```python
from build123d import *

# Parameters (mm, degrees)
F0_W      = 76.2
F0_H      = 76.2
F1_DEPTH  = 19.05
F2_R      = 25.4
F3_DEPTH  = 76.2
F5_W      = 76.2
F5_H      = 76.2
F5_R      = 25.4
F4_R      = 25.4
F6_DEPTH  = 19.05
F8_DEPTH  = 114.301
F9_R      = 6.35
F10_R     = 6.35
F11_DEPTH = 25.4
F12_R     = 6.35
F13_DEPTH = 114.301


with BuildPart() as f1:
    # F0 (on Front) → F1 (new body)
    with BuildSketch(Plane.XZ):
        with Locations((0, -0.0663684971)):
            Rectangle(F0_W, F0_H)
    extrude(amount=F1_DEPTH)

    # F2 (on face) → F3 (join)
    with BuildSketch(Plane.XZ.offset(19.05)):
        Circle(F2_R)
    extrude(amount=F3_DEPTH)

    # F5 (on face) + F4 (on face) → F6 (join)
    with BuildSketch(Plane.XZ.offset(95.25)):
        with Locations((-0.1962948591, 0.8762047957)):
            Rectangle(F5_W, F5_H)
        Circle(F5_R, mode=Mode.SUBTRACT)
    with BuildSketch(Plane.XZ.offset(95.25)):
        Circle(F4_R)
    extrude(amount=F6_DEPTH)

    # F7 (on face) → F8 (cut, through all)
    with BuildSketch(Plane.XZ.offset(114.3)):
        with BuildLine():
            Line((-0.196411438, 0.8763213746), (-13.1261387718, 13.8060487085))
            ThreePointArc((-13.1261387718, 13.8060487085), (-19.0399198266, 0.6196394072), (-13.9960272385, -12.9233788747))
            Line((-13.9960272385, -12.9233788747), (-0.196411438, 0.8763213746))
        make_face()
        with BuildLine():
            Line((13.8060487085, -13.1261387718), (-0.196411438, 0.8763213746))
            Line((-0.196411438, 0.8763213746), (-13.9960272385, -12.9233788747))
            ThreePointArc((-13.9960272385, -12.9233788747), (-0.1389275151, -19.0494934092), (13.8060487085, -13.1261387718))
        make_face()
        with BuildLine():
            Line((12.923293224, 13.9961063245), (-0.196411438, 0.8763213746))
            Line((-0.196411438, 0.8763213746), (13.8060487085, -13.1261387718))
            ThreePointArc((13.8060487085, -13.1261387718), (17.690502083, -7.067434899), (19.05, 0))
            ThreePointArc((19.05, 0), (17.4512354279, 7.6391676275), (12.923293224, 13.9961063245))
        make_face()
        with BuildLine():
            ThreePointArc((12.923293224, 13.9961063245), (-0.138985803, 19.049492984), (-13.1261387718, 13.8060487085))
            Line((-13.1261387718, 13.8060487085), (-0.196411438, 0.8763213746))
            Line((-0.196411438, 0.8763213746), (12.923293224, 13.9961063245))
        make_face()
    extrude(amount=-F8_DEPTH, mode=Mode.SUBTRACT)

    # F9 (on face) + F10 (on face) → F11 (cut)
    with BuildSketch(Plane.XZ.offset(114.3)):
        with Locations((28.3787051409, -27.6987952043)):
            Circle(F9_R)
        with Locations((-28.7712948591, 29.4512047957)):
            Circle(F9_R)
        with Locations((-28.7712948591, -27.6987952043)):
            Circle(F9_R)
    with BuildSketch(Plane.XZ.offset(114.3)):
        with Locations((28.3787051409, 29.4512047957)):
            Circle(F10_R)
    extrude(amount=-F11_DEPTH, mode=Mode.SUBTRACT)

    # F12 (on face) → F13 (cut, through all)
    with BuildSketch(Plane(origin=(0, 0, 0), x_dir=(-1, 0, 0), z_dir=(0, 1, 0))):
        with Locations((28.575, -28.6413684971)):
            Circle(F12_R)
        with Locations((28.575, 28.5086315029)):
            Circle(F12_R)
        with Locations((-28.575, 28.5086315029)):
            Circle(F12_R)
        with Locations((-28.575, -28.6247763728)):
            Circle(F12_R)
    extrude(amount=-F13_DEPTH, mode=Mode.SUBTRACT)


solid = f1.part
```
The listing builds one solid part. Answer for the finished solid, in the listing's coordinates (mm). A direction names the side the tool comes from. Give positions to 0.01 mm unless a question says otherwise; leave off trailing zeros. Order: outer loops, then holes, each group sorted by start corner. A loop starts at its lowest first (then second) coordinate and runs counter-clockwise, first axis right, second up. Notation, with made-up numbers: (50.25, 66.25) -> (81.25, 66.25) arc R28 cw to (81.25, 96.25) -> close; hole circle Ø3 at (-15.5, 20). An arc over 180 degrees is marked (long way). Write each question's results on one line, items separated by ' | '.
Q1. Straight lines are drawn through the part: probe 1 along Y at (x, z) = (26.5, -13.5); probe 2 along Z at (x, y) = (30.5, -8); probe 3 along Z at (x, y) = (3.5, -39). For each, find the intervals that lie inside material, in ascending order. Write a range as from..to.
Checked values:
probe 1: y = -114.3..-95.25, -19.05..0 | probe 2: z = -38.17..-34.68, -22.57..22.46, 34.56..38.03 | probe 3: z = -25.16..-18.73, 18.73..25.16
Q2. The part is cut by section B-B, the plane z = -6.5. Give the vertices of the cut face in (x, y).
Checked values:
outline: (-38.3, -114.3) -> (-17.91, -114.3) -> (-17.91, 0) -> (-38.1, 0) -> (-38.1, -19.05) -> (-24.55, -19.05) -> (-24.55, -95.25) -> (-38.3, -95.25) -> close; (17.91, -114.3) -> (37.9, -114.3) -> (37.9, -95.25) -> (24.55, -95.25) -> (24.55, -19.05) -> (38.1, -19.05) -> (38.1, 0) -> (17.91, 0) -> close
Q3. The part is cut by section D-D, the plane x = 29. Give the vertices of the cut face in (y, z), and give its area (3 significant figures).
Checked values:
outline: (-114.3, -37.22) -> (-95.25, -37.22) -> (-95.25, -34.96) -> (-114.3, -34.96) -> close; (-114.3, -21.38) -> (-95.25, -21.38) -> (-95.25, 22.17) -> (-114.3, 22.17) -> close; (-114.3, 35.77) -> (-95.25, 35.77) -> (-95.25, 38.98) -> (-114.3, 38.98) -> close; (-19.05, -38.17) -> (0, -38.17) -> (0, -34.96) -> (-19.05, -34.96) -> close; (-19.05, -22.29) -> (0, -22.29) -> (0, 22.17) -> (-19.05, 22.17) -> close; (-19.05, 34.84) -> (0, 34.84) -> (0, 38.03) -> (-19.05, 38.03) -> close | area: 1,900 mm^2
Q4. The part is cut by section A-A, the plane x = 0. Give the vertices of the cut face in (y, z).
Checked values:
outline: (-114.3, -37.22) -> (-95.25, -37.22) -> (-95.25, -25.4) -> (-19.05, -25.4) -> (-19.05, -38.17) -> (0, -38.17) -> (0, -19.05) -> (-114.3, -19.05) -> close; (-114.3, 19.05) -> (0, 19.05) -> (0, 38.03) -> (-19.05, 38.03) -> (-19.05, 25.4) -> (-95.25, 25.4) -> (-95.25, 38.98) -> (-114.3, 38.98) -> close
Q5. Determine the mould class of faces 1 (the face through (-9, 0, 17)), 2 (the face through (27.205, -104.908, -21.458)), 3 (the face through (-5.506, -56.617, -24.796)) for opening direction Y: pulls with the +Y half, pulls with the -Y half, needs draft (parallel to the pull), parting line crosses it, or undercut.
Checked values:
face 1: pulls with the +Y half | face 2: needs draft | face 3: undercut
Q6. The part is cut by section C-C, the plane y = -42.5. Give the vertices of the cut face in (x, z), and give its area (3 significant figures).
Checked values:
outline: circle Ø50.8 at (0, 0); hole circle Ø38.1 at (0, 0) | area: 887 mm^2
Q7. Each of these flat-tipped pins is pushed along its axis until it touches: P1, Ø9.5, axis at x = -11, y = -7, coming from the +Z side; P2, Ø11.5, axis at x = 28.58, z = -28.62, coming from the +Y side; P3, Ø5.5, axis at y = -106.5, z = 4, coming from the +X side; P4, Ø16.5, axis at x = 28.58, z = 28.51, coming from the +Y side. Where does it stop, or does it pass through?
Checked values:
P1: stops at z = 38.03 | P2: passes through | P3: stops at x = 37.9 | P4: stops at y = 0
Q8. Which of the six approach directions +Z, -Z, +X, -X, +Y, -Y give full straight-line access (tool end or side, diameter ignored) to faces 4 (the face through (-1, -9, 38.034)), 5 (the face through (-1, -95.25, 27)), 6 (the face through (-38.1, -9, -1))?
Checked values:
face 4: +Z, +X, -X, +Y | face 5: none | face 6: +Z, -Z, -X, +Y
